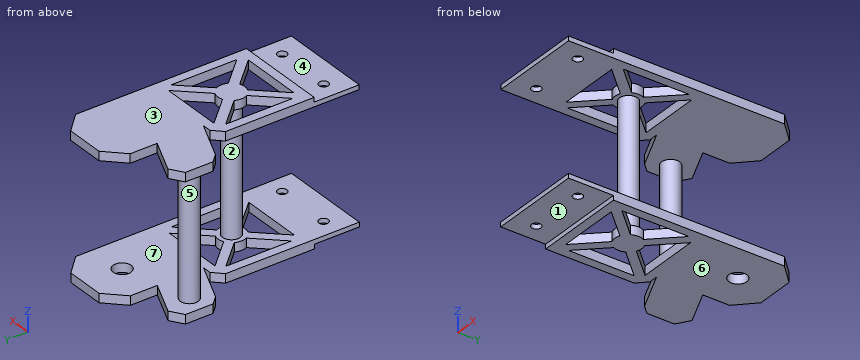
Autodesk Inventor part; units mm, degrees
ref_plane "YZ Plane" through (0, 0, 0) normal (1, 0, 0) x (0, 1, 0)
ref_plane "XZ Plane" through (0, 0, 0) normal (0, 1, 0) x (-1, 0, 0)
ref_plane "XY Plane" through (0, 0, 0) normal (0, 0, 1) x (1, 0, 0)
sketch "Esquisse2" plane through (0, 0, 0) normal (0, 0, 1) x (1, 0, 0)
  line L0 (0, 0) -> (41.5, 0)
  line L1 (41.5, 0) -> (41.5, -41.5)
  line L2 (0, 0) -> (41.5, -41.5) construction
  circle A0 centre (20.7915, -20.7085) radius 5
  line L3 (0, -25) -> (-20.4662, -16.0249)
  line L4 (-27.4743, -20.6039) -> (-27.4743, -35.9516)
  line L5 (-27.4743, -35.9516) -> (-23.1441, -40.4516)
  line L6 (0, 0) -> (0, -25)
  line L7 (-23.1441, -40.4516) -> (0, -50.6933)
  line L8 (-20.4662, -16.0249) -> (-27.4743, -20.6039)
  line L9 (41.5, -41.5) -> (41.5, -50.6933)
  line L10 (0, -50.6933) -> (-5, -50.6933)
  line L11 (-10, -55.6933) -> (-10, -130)
  line L12 (-10, -130) -> (41.5, -130)
  line L13 (41.5, -130) -> (41.5, -50.6933)
  line L14 (-5, -50.6933) -> (-10, -55.6933)
  point P0 (-10, -50.6933)
  dimension "d0" = 41.5
  dimension "d1" = 41.5
  dimension "d2" = 10
  dimension "d32" = 25
  dimension "d45" = 10
  dimension "d46" = 5
  dimension "d47" = 5
  dimension "d48" = 130
extrude "Extrusion3" add sketch "Esquisse2" along normal blind 5
sketch "Esquisse4" plane through (0, 0, 5) normal (0, 0, 1) x (1, 0, 0)
  circle A0 centre (-17.0573, -30.35) radius 5
  line L0 (0, -25) -> (-20.4662, -16.0249)
  point P0 (0, 0)
  dimension "d53" = 10
  dimension "d54" = 11.75
extrude "Extrusion4" add sketch "Esquisse4" along normal blind 70
sketch "Esquisse5" plane through (-17.0573, -30.35, 75) normal (0, 0, 1) x (1, 0, 0)
  line L0 (17.0722, 30.4073) -> (58.5722, 30.4073)
  line L1 (58.5722, 30.4073) -> (58.5722, -11.0927)
  line L2 (17.0722, 5.4073) -> (-3.394, 14.3825)
  line L3 (-10.4021, 9.8034) -> (-10.4021, -5.5443)
  line L4 (-10.4021, -5.5443) -> (-6.072, -10.0443)
  line L5 (17.0722, 30.4073) -> (17.0722, 5.4073)
  line L6 (-6.072, -10.0443) -> (17.0722, -20.2859)
  line L7 (-3.394, 14.3825) -> (-10.4021, 9.8034)
  line L8 (58.5722, -11.0927) -> (58.5722, -20.2859)
  line L9 (17.0722, -20.2859) -> (12.0722, -20.2859)
  line L10 (7.0722, -25.2859) -> (7.0722, -99.5927)
  line L11 (7.0722, -99.5927) -> (58.5722, -99.5927)
  line L12 (58.5722, -99.5927) -> (58.5722, -20.2859)
  line L13 (12.0722, -20.2859) -> (7.0722, -25.2859)
  point P0 (17.0573, 30.35)
  point P1 (7.0722, -20.2859)
  dimension "d57" = 41.5
  dimension "d58" = 41.5
  dimension "d60" = 25
  dimension "d61" = 10
  dimension "d62" = 5
  dimension "d63" = 5
  dimension "d64" = 130
chamfer "Chanfrein7" distance 10 angle 45 1 edges at (0, 0, 2.5)
chamfer "Chanfrein8" distance 10 angle 45 1 edges at (41.5, 0, 2.5)
extrude "Extrusion6" add sketch "Esquisse5" along normal blind 5
chamfer "Chanfrein9" distance 10 angle 45 1 edges at (41.5149, 0.0573, 77.5)
chamfer "Chanfrein10" distance 10 angle 45 1 edges at (0.0149, 0.0573, 77.5)
sketch "Esquisse6" plane through (0, 0, 0) normal (0, 0, -1) x (-1, 0, 0)
  line L0 (-41.5, -130) -> (9.9851, -130)
  line L1 (10, -105) -> (-41.5, -105)
  line L2 (-41.5, -105) -> (-41.5, -130)
  line L3 (9.7923, -105) -> (10, -105)
  line L4 (10, -130) -> (-41.5, -130)
  line L5 (9.8887, -130) -> (10, -130)
  line L6 (10, -130) -> (10, -55.6933)
  line L7 (10, -105) -> (10, -130)
  point P0 (0, 0)
  dimension "d87" = 25
extrude "Extrusion7" cut sketch "Esquisse6" against normal blind 2.5
sketch "Esquisse7" plane through (0, 0, 2.5) normal (0, 0, -1) x (-1, 0, 0)
  circle A0 centre (-31.5, -117.5) radius 2.6
  line L0 (-41.5, -130) -> (-41.5, -105)
  line L1 (-41.5, -105) -> (10, -105)
  circle A1 centre (-0.0149, -117.5) radius 2.6
  line L2 (9.9851, -105) -> (9.9851, -130)
  point P0 (0, 0)
  dimension "d96" = 5.2
  dimension "d97" = 10
  dimension "d98" = 12.5
  dimension "d99" = 5.2
  dimension "d100" = 10
extrude "Extrusion8" cut sketch "Esquisse7" against normal blind 2.5
sketch "Esquisse8" plane through (-17.0573, -30.35, 80) normal (0, 0, 1) x (1, 0, 0)
  line L0 (58.5573, -99.65) -> (58.5573, 20.35)
  line L1 (58.5573, -99.5927) -> (58.5573, -99.65)
  line L2 (7.0722, -99.65) -> (7.0722, -99.5927)
  line L3 (58.5722, -99.5927) -> (7.0722, -99.5927)
  line L4 (58.5722, -99.5927) -> (7.0722, -99.5927)
  line L5 (7.0722, -99.5927) -> (7.0722, -74.5927)
  line L6 (7.0722, -74.5927) -> (58.5722, -74.5927)
  line L7 (58.5722, -74.5927) -> (58.5722, -99.5927)
  point P0 (17.0573, 30.35)
  dimension "d103" = 25
extrude "Extrusion10" cut sketch "Esquisse8" against normal blind 2.5
sketch "Esquisse9" plane through (-17.0573, -30.35, 77.5) normal (0, 0, 1) x (1, 0, 0)
  circle A0 centre (17.0722, -87.15) radius 2.6
  circle A1 centre (17.0722, -87.15) radius 2.6
  circle A2 centre (48.5573, -87.15) radius 2.6
  circle A3 centre (48.5573, -87.15) radius 2.6
  point P0 (17.0573, 30.35)
extrude "Extrusion11" cut sketch "Esquisse9" against normal blind 2.5
sketch "Esquisse10" plane through (0, 0, 0) normal (0, 0, -1) x (-1, 0, 0)
  line L0 (0, -50.6933) -> (9.9851, -50.6933) construction
  line L1 (9.9851, -50.6933) -> (9.9851, -105) construction
  line L2 (0, -50.6933) -> (-41.5, -50.6933) construction
  line L3 (-41.5, -10) -> (-41.5, -105) construction
  line L4 (-41.5, -105) -> (-41.5, -50.6933) construction
  line L5 (-31.0711, -55.6933) -> (4.9851, -55.6933)
  line L6 (4.9851, -55.6933) -> (4.9851, -100)
  line L7 (-31.0711, -55.6933) -> (-36.5, -55.6933)
  line L8 (-36.5, -55.6933) -> (-36.5, -59.2233) construction
  line L9 (-36.5, -55.6933) -> (-33.2298, -55.6933) construction
  line L10 (-41.5, -105) -> (9.9851, -105) construction
  line L11 (-36.5, -55.6933) -> (-36.5, -100)
  line L12 (-36.5, -100) -> (4.9851, -100)
  line L13 (-36.5, -55.6933) -> (4.9851, -100) construction
  line L14 (4.9851, -55.6933) -> (-36.5, -100) construction
  circle A0 centre (-15.7574, -77.8466) radius 7.5
  line L15 (-36.5, -100) -> (-36.5, -96.47) construction
  line L16 (-36.5, -100) -> (-32.97, -100) construction
  line L17 (-32.97, -100) -> (-18.6905, -84.7493)
  line L18 (-9.0624, -74.4663) -> (4.9851, -59.4633)
  line L19 (-12.5184, -71.0821) -> (1.8904, -55.6933)
  line L20 (-12.665, -84.6794) -> (1.6799, -100)
  line L21 (-8.98, -81.0585) -> (4.9851, -95.9735)
  line L22 (-36.5, -59.2233) -> (-36.5, -96.6948)
  line L23 (-32.7299, -55.6933) -> (1.8904, -55.6933)
  line L24 (4.9851, -59.4633) -> (4.9851, -95.9735)
  line L25 (1.6799, -100) -> (-32.97, -100)
  line L26 (-32.7299, -55.6933) -> (-18.5171, -70.8728)
  line L27 (-36.5, -59.4633) -> (-22.4232, -74.409)
  line L28 (-36.5, -96.6948) -> (-22.2945, -81.5231)
  point P0 (0, 0)
  point P1 (9.9851, -104.9427)
  point P2 (-41.5149, -104.9427)
  dimension "d57" = 41.5
  dimension "d58" = 41.5
  dimension "d60" = 25
  dimension "d61" = 10
  dimension "d62" = 5
  dimension "d63" = 5
  dimension "d64" = 130
  dimension "d118" = 15
  dimension "d110" = 5
  dimension "d111" = 5
  dimension "d116" = 5
  dimension "d117" = 5
extrude "Extrusion12" cut sketch "Esquisse10" against normal blind 5 contours L5 L19 A0 L26 L7 | L6 L21 A0 L18 | A0 L28 L11 L27 | A0 L20 L12 L17
sketch "Esquisse11" plane through (-17.0573, -30.35, 80) normal (0, 0, 1) x (1, 0, 0)
  line L0 (48.5721, -20.2859) -> (58.5722, -20.2859) construction
  line L1 (58.5722, -20.2859) -> (58.5722, -74.5927) construction
  line L2 (48.5721, -20.2859) -> (7.0573, -20.2859) construction
  line L3 (17.501, -25.2859) -> (53.5722, -25.2859)
  line L4 (53.5722, -25.2859) -> (53.5722, -69.5927)
  line L5 (17.501, -25.2859) -> (12.0573, -25.2859)
  line L6 (12.0573, -25.2859) -> (12.0573, -28.8108) construction
  line L7 (12.0573, -25.2859) -> (15.3423, -25.2859) construction
  line L8 (7.0573, -74.5927) -> (58.5722, -74.5927) construction
  line L9 (12.0573, -25.2859) -> (12.0573, -69.5927)
  line L10 (12.0573, -69.5927) -> (53.5722, -69.5927)
  line L11 (12.0573, -25.2859) -> (53.5722, -69.5927) construction
  line L12 (53.5722, -25.2859) -> (12.0573, -69.5927) construction
  circle A0 centre (32.8147, -47.4393) radius 7.5
  line L13 (12.0573, -69.5927) -> (12.0573, -66.0575) construction
  line L14 (12.0573, -69.5927) -> (15.6035, -69.5927) construction
  line L15 (15.6035, -69.5927) -> (29.8797, -54.3412)
  line L16 (39.5079, -44.0553) -> (53.5722, -29.0303)
  line L17 (36.0535, -40.6747) -> (50.4623, -25.2859)
  line L18 (35.9101, -54.2708) -> (50.2563, -69.5927)
  line L19 (39.5942, -50.647) -> (53.5722, -65.5758)
  line L20 (12.0573, -28.8108) -> (12.0573, -66.2913)
  line L21 (15.8474, -25.2859) -> (50.4623, -25.2859)
  line L22 (53.5722, -29.0303) -> (53.5722, -65.5758)
  line L23 (50.2563, -69.5927) -> (15.6035, -69.5927)
  line L24 (15.8474, -25.2859) -> (30.0589, -40.464)
  line L25 (12.0573, -29.0404) -> (26.1489, -44.0018)
  line L26 (12.0573, -66.2913) -> (26.2734, -51.1082)
  line L27 (58.5722, -74.5927) -> (58.5722, 20.4073)
  line L28 (7.0722, -74.5927) -> (58.5722, -74.5927)
  line L29 (17.0722, -20.2859) -> (12.0722, -20.2859)
  line L30 (7.0722, -25.2859) -> (7.0722, -74.5927)
  line L31 (12.0573, -29.0404) -> (12.0573, -66.2913)
  point P0 (17.0573, 30.35)
  point P1 (0, 0)
  point P2 (58.5572, -74.5302)
  point P3 (7.0572, -74.5302)
  dimension "d127" = 15
  dimension "d123" = 5
  dimension "d124" = 5
  dimension "d126" = 5
  dimension "d128" = 0
  dimension "d129" = 0
  dimension "d130" = 0
extrude "Extrusion13" cut sketch "Esquisse11" against normal blind 5 contours L3 L17 A0 L24 L5 | L4 L19 A0 L16 | A0 L26 L9 L25 | A0 L18 L10 L15
sketch "Esquisse14" plane through (-17.0573, -30.35, 75) normal (0, 0, -1) x (-1, 0, 0)
  arc A0 (-39.5079, -44.0553) -> (-39.5942, -50.647) centre (-32.8147, -47.4393) ccw
  circle A1 centre (-32.8147, -47.4393) radius 5
  point P0 (-17.0573, 30.35)
  dimension "d136" = 10
extrude "Extrusion14" add sketch "Esquisse14" along normal blind 70
equation "\"d63\" = d62"
properties part number "Forearm1 v2" material "Plastique ABS"
Read the model definition and answer for the solid it produces. Units are mm, in the model's axes. Face numbers are marked on the shaded views. A direction names the side the tool comes from. Give positions to 0.01 mm unless a question says otherwise; leave off trailing zeros. Order: outer loops, then holes, each group sorted by start corner. A loop starts at its lowest first (then second) coordinate and runs counter-clockwise, first axis right, second up. Notation, with made-up numbers: (36.5, 28.5) -> (92.5, 28.5) arc R22 cw to (92.5, 39.5) -> close; hole circle Ø10 at (-33, -12). An arc over 180 degrees is marked (long way). One line per item, written item: value. Start each with the question number.
(1) For a pull along Z with two mould halves and no side action, classify the marked faces 4, 5, 6 and 7 as released by +Z, released by -Z, zero draft, split by the parting line, or undercut.
(2) The part is cut by section C-C (z = 59). Determine the outline of the cut face in (x, y).
(3) Straight lines are drawn through the part: L1, parallel to Z at x = 22.5, y = -39; L2, parallel to Y at x = 12, z = 76.5; L3, parallel to Z at x = 4, y = -123. For each, find the intervals that lie inside material, in ascending order.
(4) The part is cut by section D-D (y = -65.5). State how many separate pieces and enclosed holes the cut face has, and give its area (3 significant figures).
(5) Flat-ended cylindrical pins translate along their axes: P1, Ø4, axis at y = -77.5, z = 15.5, coming from the -X side; P2, Ø7.5, axis at x = 8, y = -114.5, coming from the -Z side; P3, Ø3, axis at x = -15, z = 51.5, coming from the -Y side; P4, Ø4.5, axis at x = 0.01, y = -117.5, coming from the -Z side. Find the tip coordinate at first contact, or state that the pin passes through.
(6) A tool of negligible diameter and unlimited length cuts with its end or side. For the marked faces 1, 2 and 3, from which of +Z, -Z, +X, -X, +Y, -Y can it reach the whole face along a straight path? Write none if from no direction.
(7) The part is cut by section B-B (y = -37.5). Determine the outline of the cut face in (x, z), and give its area (3 significant figures).
(8) The part is cut by section A-A (y = -117.5). Determine the outline of the cut face in (x, z).
Taken from the geometry:
1. face 4: released by +Z
1. face 5: undercut
1. face 6: released by -Z
1. face 7: undercut
2. outline: circle Ø10 at (-17.06, -30.35); circle Ø10 at (15.76, -77.79)
3. L1: 0 to 5, 75 to 80
3. L2: -129.94 to -99.94, -85.57 to -69.74, -55.64 to 0.06
3. L3: 2.5 to 5, 75 to 77.5
4. separate pieces: 8
4. enclosed holes: 0
4. area: 239 mm^2
5. P1: x = 10.76
5. P2: z = 2.5
5. P3: y = -35.32
5. P4: through
6. face 1: -Z, +X, -X, -Y
6. face 2: none
6. face 3: +Z, +X, -X, +Y, -Y
7. outline: (-25.98, 0) -> (41.5, 0) -> (41.5, 5) -> (-25.98, 5) -> close; (-25.91, 75) -> (41.51, 75) -> (41.51, 80) -> (-25.91, 80) -> close
7. area: 675 mm^2
8. outline: (-10, 2.5) -> (-2.59, 2.5) -> (-2.59, 5) -> (-10, 5) -> close; (-9.99, 75) -> (-2.59, 75) -> (-2.59, 77.5) -> (-9.99, 77.5) -> close; (2.61, 2.5) -> (28.9, 2.5) -> (28.9, 5) -> (2.61, 5) -> close; (2.61, 75) -> (28.9, 75) -> (28.9, 77.5) -> (2.61, 77.5) -> close; (34.1, 2.5) -> (41.5, 2.5) -> (41.5, 5) -> (34.1, 5) -> close; (34.1, 75) -> (41.51, 75) -> (41.51, 77.5) -> (34.1, 77.5) -> close
